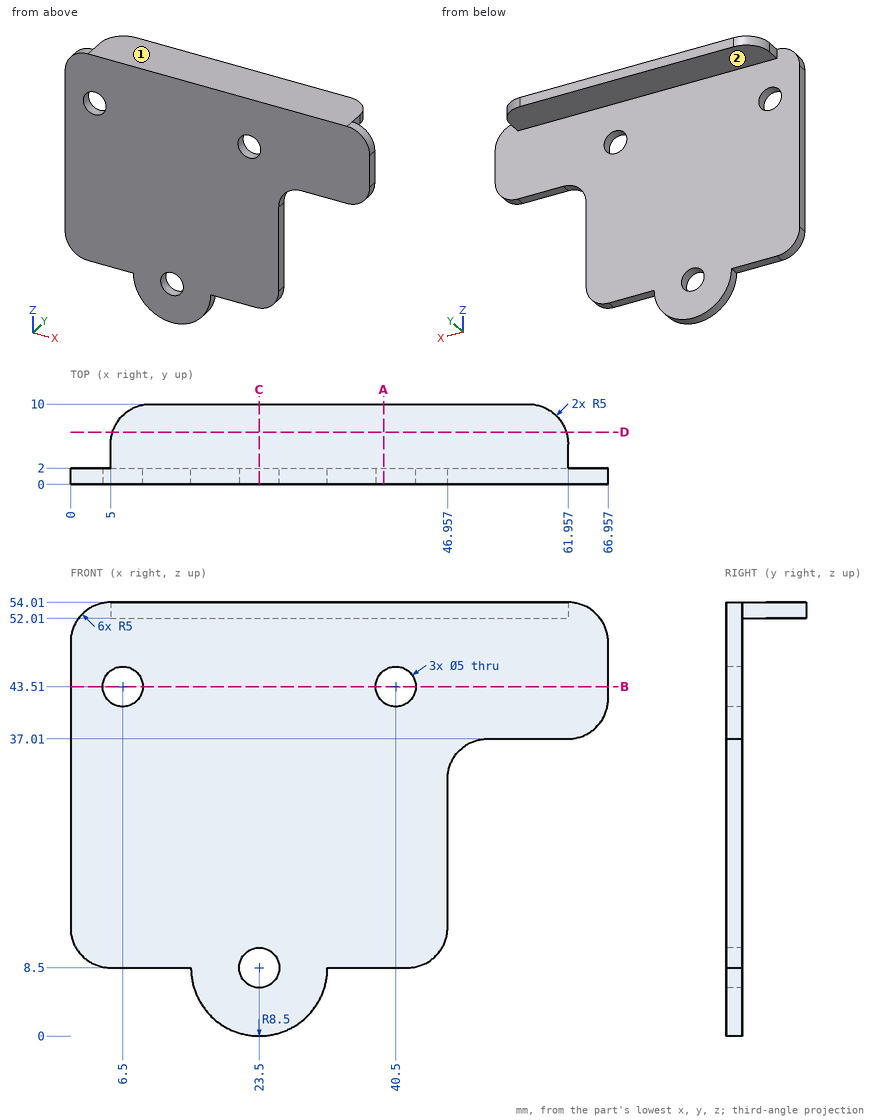
Verification items for this drawing (mm, ordinates from the low corner). A direction names the side the tool comes from. Give positions to 0.01 mm unless a question says otherwise; leave off trailing zeros. Loops run counter-clockwise (first coordinate to the right, second up) from the corner with the lowest first, then second, coordinate; pieces in that order, holes last. Notation, with made-up numbers: M -20.5,15.5 L 27.5,15.5 A24 cw 27.5,43.5 Z; hole C -36,-21.5 d1. An arc over 180 degrees is marked long. Write item = value, one per line. Start each with the question number.
1. Go/stop test with flat-tipped pins: P1, Ø16, axis at x = 41, z = 18.5, coming from the +Y side; P2, Ø1.6, axis at y = 4, z = 53, coming from the -X side; P3, Ø4.5, axis at x = 23.5, z = 8.5, coming from the -Y side; P4, Ø2, axis at y = 1, z = 20.5, coming from the +X side. Record where each tip stops, or that it passes through.
2. Section check C-C, the plane x = 23.5. Enter the section's corners in (y, z), plus the area to 3 significant figures.
3. Section check B-B, the plane z = 43.51. Enter the section's corners in (x, y), plus the area to 3 significant figures.
4. Section check A-A, the plane x = 39. Enter the section's corners in (y, z).
5. Section check D-D, the plane y = 6.5. Enter the section's corners in (x, z), plus the area to 3 significant figures.
6. Thickness scan on probe 1 along X at (y, z) = (1.4, 43.51); probe 2 along Z at (x, y) = (23.5, 1.5); probe 3 along Z at (x, y) = (6.5, 0.75). Record the ranges inside material, lowest first.
7. Tool access check on the marked faces 1 and 2. Record the directions out of +Z, -Z, +X, -X, +Y, -Y that give a thin tool (end or side, any length) a straight path to the whole face; none if there is none.
Values follow:
q1.P1 = 2
q1.P2 = 5
q1.P3 = through
q1.P4 = 46.96
q2.outline = M 0,0 L 2,0 L 2,6 L 0,6 Z; M 0,11 L 2,11 L 2,52.01 L 10,52.01 L 10,54.01 L 0,54.01 Z
q2.area = 114 mm^2
q3.outline = M 0,0 L 4,0 L 4,2 L 0,2 Z; M 9,0 L 38,0 L 38,2 L 9,2 Z; M 43,0 L 66.96,0 L 66.96,2 L 43,2 Z
q3.area = 114 mm^2
q4.outline = M 0,8.5 L 2,8.5 L 2,41.51 L 0,41.51 Z; M 0,45.51 L 2,45.51 L 2,52.01 L 10,52.01 L 10,54.01 L 0,54.01 Z
q5.outline = M 5.23,52.01 L 61.73,52.01 L 61.73,54.01 L 5.23,54.01 Z
q5.area = 113 mm^2
q6.probe_1 = 0 to 4, 9 to 38, 43 to 66.96
q6.probe_2 = 0 to 6, 11 to 54.01
q6.probe_3 = 8.5 to 41.01, 46.01 to 54.01
q7.face_1 = +Z, +X, -X, +Y, -Y
q7.face_2 = -Z, +X, -X, +Y
